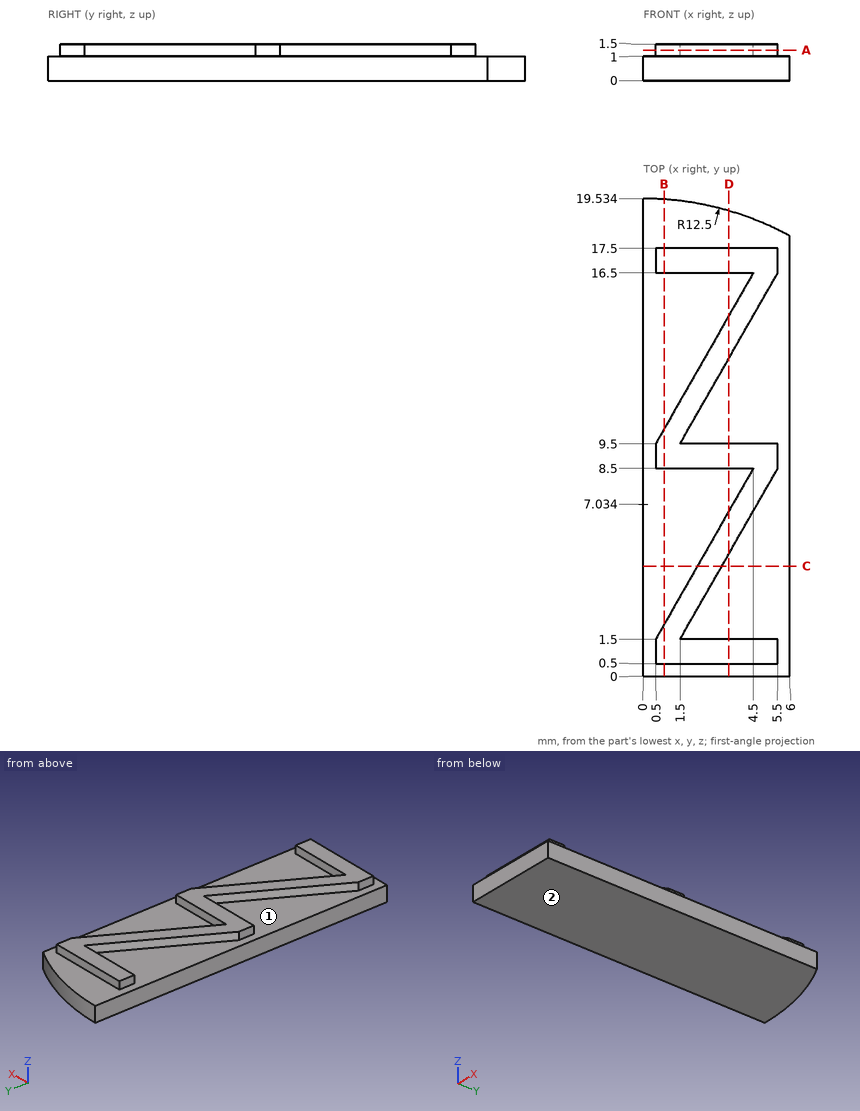
Source: three-view drawing plus pictorial views. Frame: mm from the lowest corner of the part. Give positions to 0.01 mm unless a question says otherwise; leave off trailing zeros. Order: outer loops, then holes, each group sorted by start corner. A loop starts at its lowest first (then second) coordinate and runs counter-clockwise, first axis right, second up. Notation, with made-up numbers: M -38,-5.5 L -21,-5.5 A20 ccw -21,19.5 Z; hole C 88,-32 d6. An arc over 180 degrees is marked long. Return JSON: item names as keys, results as strings.
1) Section query A-A on z = 1.25. Output: boundary loops of the cut face in (x, y).
Taken from the geometry:
{"outline": "M 0.5,0.5 L 5.5,0.5 L 5.5,1.5 L 1.5,1.5 L 5.5,8.5 L 5.5,9.5 L 1.5,9.5 L 5.5,16.5 L 5.5,17.5 L 0.5,17.5 L 0.5,16.5 L 4.5,16.5 L 0.5,9.5 L 0.5,8.5 L 4.5,8.5 L 0.5,1.5 Z"}
2) Contact query for flat-ended pins moving along their axis: pin 1 (0.6 mm diameter, centred on x = 3, z = 1, fed in from +Y); pin 2 (0.6 mm diameter, centred on y = 9, z = 1.5, fed in from -X); pin 3 (1.8 mm diameter, centred on x = 4, y = 11.5, fed in from +Z). Output: stop coordinate, or through.
Taken from the geometry:
{"pin 1": "stops at y = 19.24", "pin 2": "stops at x = 0.5", "pin 3": "stops at z = 1"}
3) Section query C-C on y = 4.5. Output: boundary loops of the cut face in (x, z).
Taken from the geometry:
{"outline": "M 0,0 L 6,0 L 6,1 L 3.21,1 L 3.21,1.5 L 2.21,1.5 L 2.21,1 L 0,1 Z"}
4) Line query: L1, parallel to Y at x = 3, z = 1.1 (1 decimal); L2, parallel to Y at x = 3.75, z = 1.4; L3, parallel to Z at x = 4.15, y = 13.5. Output: solid intervals per line, ascending. Write a range as [from, to].
Taken from the geometry:
{"L1": "y = [0.5, 1.5], [4.1, 5.9], [8.5, 9.5], [12.1, 13.9], [16.5, 17.5]", "L2": "y = [0.5, 1.5], [5.44, 7.19], [8.5, 9.5], [13.44, 15.19], [16.5, 17.5]", "L3": "z = [0, 1]"}
5) Mould query, pull axis Y, two halves, no side actions, for the marked faces 1 and 2. Classes: released by +Y, released by -Y, zero draft, split by the parting line, or undercut.
Taken from the geometry:
{"face 1": "undercut", "face 2": "zero draft"}
6) Section query B-B on x = 0.85. Output: boundary loops of the cut face in (y, z) (1 decimal), and give its area (3 significant figures).
Taken from the geometry:
{"outline": "M 0,0 L 19.5,0 L 19.5,1 L 17.5,1 L 17.5,1.5 L 16.5,1.5 L 16.5,1 L 10.1,1 L 10.1,1.5 L 8.5,1.5 L 8.5,1 L 2.1,1 L 2.1,1.5 L 0.5,1.5 L 0.5,1 L 0,1 Z", "area": "21.6 mm2"}
7) Section query D-D on x = 3.5. Output: boundary loops of the cut face in (y, z).
Taken from the geometry:
{"outline": "M 0,0 L 19.03,0 L 19.03,1 L 17.5,1 L 17.5,1.5 L 16.5,1.5 L 16.5,1 L 14.75,1 L 14.75,1.5 L 13,1.5 L 13,1 L 9.5,1 L 9.5,1.5 L 8.5,1.5 L 8.5,1 L 6.75,1 L 6.75,1.5 L 5,1.5 L 5,1 L 1.5,1 L 1.5,1.5 L 0.5,1.5 L 0.5,1 L 0,1 Z"}
